Autodesk Inventor part; units mm, degrees
ref_plane "YZ Plane" through (0, 0, 0) normal (1, 0, 0) x (0, 1, 0)
ref_plane "XZ Plane" through (0, 0, 0) normal (0, 1, 0) x (-1, 0, 0)
ref_plane "XY Plane" through (0, 0, 0) normal (0, 0, 1) x (1, 0, 0)
sketch "Sketch1" plane through (0, 0, 0) normal (0, 0, 1) x (1, 0, 0)
  line L0 (0, 0) -> (30, 0)
  line L1 (30, 0) -> (30, 100)
  line L2 (30, 100) -> (0, 100)
  line L3 (0, 100) -> (0, 0)
  dimension "d0" = 30
  dimension "d1" = 100
extrude "Extrusion1" add sketch "Sketch1" along normal blind 3
sketch "Sketch2" plane through (0, 0, 3) normal (0, 0, 1) x (1, 0, 0)
  circle A0 centre (15, 85) radius 4
  line L0 (30, 0) -> (30, 100)
  line L1 (30, 100) -> (0, 100)
  point P0 (0, 0)
  dimension "d4" = 8
  dimension "d5" = 15
  dimension "d6" = 15
extrude "Extrusion2" cut sketch "Sketch2" against normal through all
properties part number "Chapa para sensor ultrassônico" material "Steel AISI 1006 85 HR"
Geometry: final body of the model. Coordinates: model frame, mm. Give positions to 0.01 mm unless a question says otherwise; leave off trailing zeros. Write each loop counter-clockwise with the first axis right and the second up, starting at its lowest first coordinate (ties: lowest second). Pieces come first, ordered by that corner, then holes.
1. Section query B-B, the plane x = 15. Return loops of the section in (y, z), then the cut area to 3 significant figures.
2. Draft query along X for faces 1 (the flat face through (30, 49, 1)), 2 (the cylindrical face through (14.133, 81.095, 1.521)), 3 (the flat face through (0, 51, 1)), 4 (the flat face through (15, 0, 1)). Return one class per face: released by +X, released by -X, zero draft, split by the parting line, or undercut.
3. Section query C-C, the plane z = 0.75. Return loops of the section in (x, y), then the cut area to 3 significant figures.
4. Line query: probe 1 along Y at (x, z) = (15, 1.45); probe 2 along Y at (x, z) = (18.5, 0.5). Output: solid intervals per line, ascending.
5. Section query A-A, the plane y = 85. Return loops of the section in (x, z), then the cut area to 3 significant figures.
Computed:
1. outline: (0, 0) - (81, 0) - (81, 3) - (0, 3) - close; (89, 0) - (100, 0) - (100, 3) - (89, 3) - close
1. area: 276 mm2
2. face 1: released by +X
2. face 2: undercut
2. face 3: released by -X
2. face 4: zero draft
3. outline: (0, 0) - (30, 0) - (30, 100) - (0, 100) - close; hole circle Ø8 at (15, 85)
3. area: 2,950 mm2
4. probe 1: y = 0 to 81, 89 to 100
4. probe 2: y = 0 to 83.06, 86.94 to 100
5. outline: (0, 0) - (11, 0) - (11, 3) - (0, 3) - close; (19, 0) - (30, 0) - (30, 3) - (19, 3) - close
5. area: 66.0 mm2
